The listing builds one solid part. Answer for the finished solid, in the listing's coordinates (mm). A direction names the side the tool comes from. Round coordinates to 2 decimals unless told otherwise and drop trailing zeros. Loops run counter-clockwise (first coordinate to the right, second up) from the corner with the lowest first, then second, coordinate; pieces in that order, holes last. Notation, with made-up numbers: M 1,44 L 17,44 A29 cw 17,66 Z; hole C 80,-28.75 d8. An arc over 180 degrees is marked long. Put each result on its own line as item: value. Start each with the question number.
(1) Straight lines are drawn through the part: line 1 (X direction, y = -3, z = 0.25); line 2 (Z direction, x = 8.75, y = -1.25); line 3 (Z direction, x = -0.25, y = 1.25). For each, find the intervals that lie inside material, in ascending order.
(2) Flat-ended cylindrical pins translate along their axes: P1, Ø2, axis at x = 5, z = 3, coming from the +Y side; P2, Ø1, axis at x = 7.5, y = 2.5, coming from the -Z side; P3, Ø3, axis at x = 10, y = 0, coming from the -Z side. Find the tip coordinate at first contact, or state that the pin passes through.
(3) Section B-B, the plane x = -2 is taken. Determine the outline of the cut face in (y, z).
(4) Which of the six approach directions +Z, -Z, +X, -X, +Y, -Y give full straight-line access (tool end or side, diameter ignored) to faces 1 (the face through (0, 1, -0.3)), 2 (the face through (-2.528, 2.535, -1.31)), 3 (the face through (-0.5, -0.4, -2.2))?
(5) Section A-A, the plane x = 9.5 is taken. Determine the outline of the cut face in (y, z), then the cut area to 3 significant figures.
Solid Edge part; units mm, degrees
sketch "Sketch1" plane through (0, 0, 0) normal (0, -1, 0) x (1, 0, 0)
  line L0 (12.5, 0) -> (12.5, 3)
  line L1 (0, 3) -> (12.5, 3)
  line L2 (0, 3) -> (0, 0)
  line L3 (0, 0) -> (12.5, 0)
revolve "RevolvedProtrusion1" add sketch "Sketch1" angle 360 about axis through (0, 0, 3) along (1, 0, 0)
sketch "Sketch2" plane through (0, 0, 3) normal (-1, 0, 0) x (0, -1, 0)
  circle A0 centre (0, 0) radius 5
extrude "Protrusion1" add sketch "Sketch2" along normal blind 0.5
sketch "Sketch3" plane through (-0.5, 0, 3) normal (-1, 0, 0) x (0, -1, 0)
  circle A0 centre (0, 0) radius 5
extrude "Protrusão_Extrudada_5" add sketch "Sketch3" along normal blind 4
sketch "Sketch4" plane through (-4.5, 0, 3) normal (-1, 0, 0) x (0, -1, 0)
  line L0 (-5, 2.8868) -> (-5, -2.8868)
  line L1 (-5, -2.8868) -> (0, -5.7735)
  line L2 (0, -5.7735) -> (5, -2.8868)
  line L3 (5, -2.8868) -> (5, 2.8868)
  line L4 (5, 2.8868) -> (0, 5.7735)
  line L5 (0, 5.7735) -> (-5, 2.8868)
extrude "Protrusão_Extrudada_8" add sketch "Sketch4" against normal blind 4
fillet "Redondo_2" radius 0.25 1 edges at (0, 0, 6)
sketch "Sketch5" plane through (0, 0, 0) normal (0, 1, 0) x (-1, 0, 0)
  line L0 (4.5, 8.7735) -> (4.05, 8.7735)
  line L1 (4.5, 8.0035) -> (4.05, 8.7735)
  line L2 (4.5, 8.7735) -> (4.5, 8.0035)
revolve "RevolvedCutout1" cut sketch "Sketch5" angle 360 about axis through (-4.5, 0, 3) along (1, 0, 0)
properties material "Polypropylene, high impact"
Recorded:
1. line 1: x = -4.5 to 0
1. line 2: z = 0.27 to 5.73
1. line 3: z = -1.84 to 7.84
2. P1: stops at y = 3
2. P2: stops at z = 0.76
2. P3: stops at z = 0
3. outline: M -5,0.11 L 0,-2.77 L 5,0.11 L 5,5.89 L 0,8.77 L -5,5.89 Z
4. face 1: +X
4. face 2: -Z, +X, -X, +Y
4. face 3: -Z, +X
5. outline: C 0,3 d6
5. area: 28.3 mm²
